Answer from the drawing. Dimensions are ordinates in mm from the lowest x, y and z of the part. A direction names the side the tool comes from. Coordinates: 2 decimals unless noted, no trailing zeros. Write each loop counter-clockwise with the first axis right and the second up, starting at its lowest first coordinate (ties: lowest second). Pieces come first, ordered by that corner, then holes. Notation, with made-up numbers: (6, 82) - (49, 82) arc R16 ccw to (49, 110) - close; hole circle Ø6 at (17, 58). An arc over 180 degrees is marked (long way). Use a Markdown table: item, result.
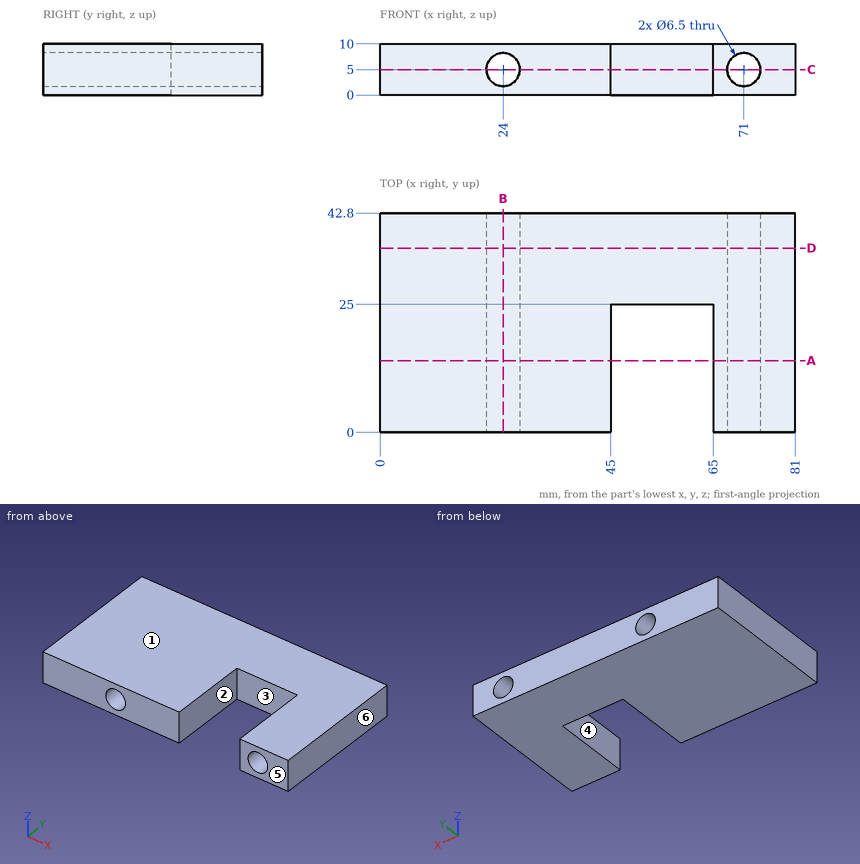
(1) For the marked faces 1 and 2, determine the directions among +Z, -Z, +X, -X, +Y, -Y from which every point of the face is accessible in a straight line to the end or side of a thin tool.
Report:
| item | result |
|---|---|
| face 1 | +Z, +X, -X, +Y, -Y |
| face 2 | +Z, -Z, -Y |
(2) A cutting plane is placed at D-D, the plane y = 36. Write down the section's boundary in (x, z).
Report:
| item | result |
|---|---|
| outline | (0, 0) - (81, 0) - (81, 10) - (0, 10) - close; hole circle Ø6.5 at (24, 5); hole circle Ø6.5 at (71, 5) |
(3) A cutting plane is placed at B-B, the plane x = 24. Write down the section's boundary in (y, z), and give its area (3 significant figures).
Report:
| item | result |
|---|---|
| outline | (0, 0) - (42.8, 0) - (42.8, 1.75) - (0, 1.75) - close; (0, 8.25) - (42.8, 8.25) - (42.8, 10) - (0, 10) - close |
| area | 150 mm² |
(4) Each of these flat-tipped pins is pushed along its axis until it touches: P1, Ø3, axis at x = 56.5, z = 3.5, coming from the -Y side; P2, Ø5, axis at y = 16, z = 4, coming from the -X side. Where does it stop, or does it pass through?
Report:
| item | result |
|---|---|
| P1 | stops at y = 25 |
| P2 | stops at x = 0 |
(5) Straight lines are drawn through the part: L1, parallel to X at y = 11, z = 5; L2, parallel to X at y = 26, z = 5; L3, parallel to X at y = 22, z = 0.5. For each, find the intervals that lie inside material, in ascending order.
Report:
| item | result |
|---|---|
| L1 | x = 0 to 20.75, 27.25 to 45, 65 to 67.75, 74.25 to 81 |
| L2 | x = 0 to 20.75, 27.25 to 67.75, 74.25 to 81 |
| L3 | x = 0 to 45, 65 to 81 |
(6) The mould has two halves that part along X. Classify the marked faces 3, 4, 5 and 6: pulls with the +X half, pulls with the -X half, needs draft (parallel to the pull), parting line crosses it, or undercut.
Report:
| item | result |
|---|---|
| face 3 | undercut |
| face 4 | undercut |
| face 5 | needs draft |
| face 6 | pulls with the +X half |
(7) A cutting plane is placed at C-C, the plane z = 5. Write down the section's boundary in (x, y), and give its area (3 significant figures).
Report:
| item | result |
|---|---|
| outline | (0, 0) - (20.75, 0) - (20.75, 42.8) - (0, 42.8) - close; (27.25, 0) - (45, 0) - (45, 25) - (65, 25) - (65, 0) - (67.75, 0) - (67.75, 42.8) - (27.25, 42.8) - close; (74.25, 0) - (81, 0) - (81, 42.8) - (74.25, 42.8) - close |
| area | 2,410 mm² |
(8) A cutting plane is placed at A-A, the plane y = 14. Write down the section's boundary in (x, z).
Report:
| item | result |
|---|---|
| outline | (0, 0) - (45, 0) - (45, 10) - (0, 10) - close; (65, 0) - (81, 0) - (81, 10) - (65, 10) - close; hole circle Ø6.5 at (24, 5); hole circle Ø6.5 at (71, 5) |
